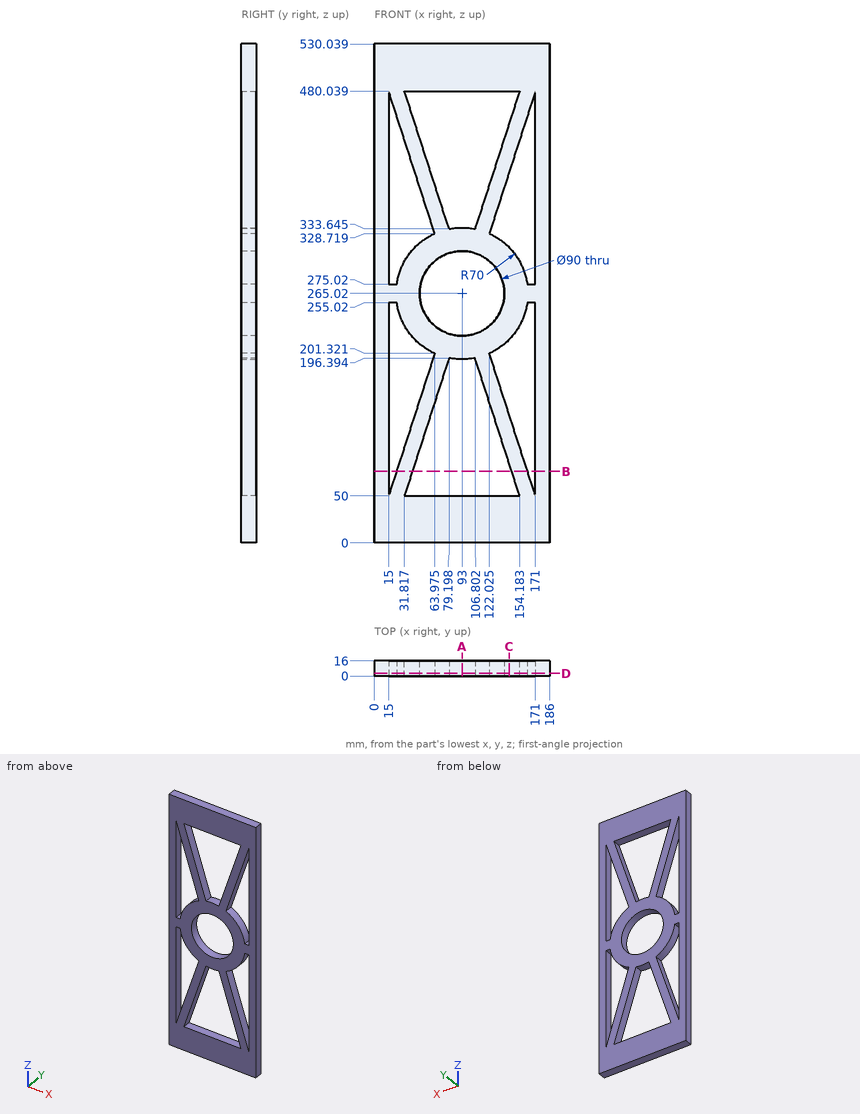
Could you check a few things on this drawing? It's one solid part, dimensions in mm from its lowest x, y, z. Coordinates: 2 decimals unless noted, no trailing zeros. Order: outer loops, then holes, each group sorted by start corner. A loop starts at its lowest first (then second) coordinate and runs counter-clockwise, first axis right, second up. Notation, with made-up numbers: M 12.25,-34.5 L 38.25,-34.5 A19 ccw 38.25,-3.5 Z; hole C -28,88.25 d8. An arc over 180 degrees is marked long. Use a Markdown table: item, result. Add a question column.
Q1. I want a section at D-D on y = 2.75. Give the number of separate pieces and of enclosed holes in the cut face, then the cut area to 3 significant figures.
Q2. I want a section at A-A on x = 93. List the corners of the cut face in (y, z) for me.
Q3. I want a section at B-B on z = 76. List the corners of the cut face in (x, y) for me (1 decimal), then the cut area to 3 significant figures.
Q4. I want a section at C-C on x = 143. List the corners of the cut face in (y, z) for me.
Q5. If I drill on L1, parallel to Z at x = 84, y = 9.5; L2, parallel to X at y = 6, z = 78.5 (1 decimal); L3, parallel to Z at x = 103, y = 8.5 (1 decimal), over which ranges is the centre line in solid material (lowest first)?
Checked values:
| question | item | result |
|---|---|---|
| 1 | separate pieces | 1 |
| 1 | enclosed holes | 7 |
| 1 | area | 50,900 mm² |
| 2 | outline | M 0,0 L 16,0 L 16,50 L 0,50 Z; M 0,195.02 L 16,195.02 L 16,220.02 L 0,220.02 Z; M 0,310.02 L 16,310.02 L 16,335.02 L 0,335.02 Z; M 0,480.04 L 16,480.04 L 16,530.04 L 0,530.04 Z |
| 3 | outline | M 0,0 L 15,0 L 15,16 L 0,16 Z; M 23.4,0 L 40.2,0 L 40.2,16 L 23.4,16 Z; M 145.8,0 L 162.6,0 L 162.6,16 L 145.8,16 Z; M 171,0 L 186,0 L 186,16 L 171,16 Z |
| 3 | area | 1,020 mm² |
| 4 | outline | M 0,0 L 16,0 L 16,50 L 0,50 Z; M 0,84.55 L 16,84.55 L 16,136.51 L 0,136.51 Z; M 0,216.03 L 16,216.03 L 16,314.01 L 0,314.01 Z; M 0,393.53 L 16,393.53 L 16,445.49 L 0,445.49 Z; M 0,480.04 L 16,480.04 L 16,530.04 L 0,530.04 Z |
| 5 | L1 | 0 to 50, 195.6 to 220.93, 309.11 to 334.44, 480.04 to 530.04 |
| 5 | L2 | 0 to 15, 24.2 to 41, 145 to 161.8, 171 to 186 |
| 5 | L3 | 0 to 50, 195.7 to 221.1, 308.9 to 334.3, 480 to 530 |
